Answer from the drawing. Dimensions are ordinates in mm from the lowest x, y and z of the part. Round coordinates to 2 decimals unless told otherwise and drop trailing zeros. Write each loop counter-clockwise with the first axis right and the second up, starting at its lowest first coordinate (ties: lowest second). Pieces come first, ordered by that corner, then holes. Notation, with made-up numbers: (5, 56.25) - (56, 56.25) arc R10 ccw to (56, 72.25) - close; hole circle Ø5 at (80, -24). An arc over 180 degrees is marked (long way). Answer in a Markdown table with one row per item.
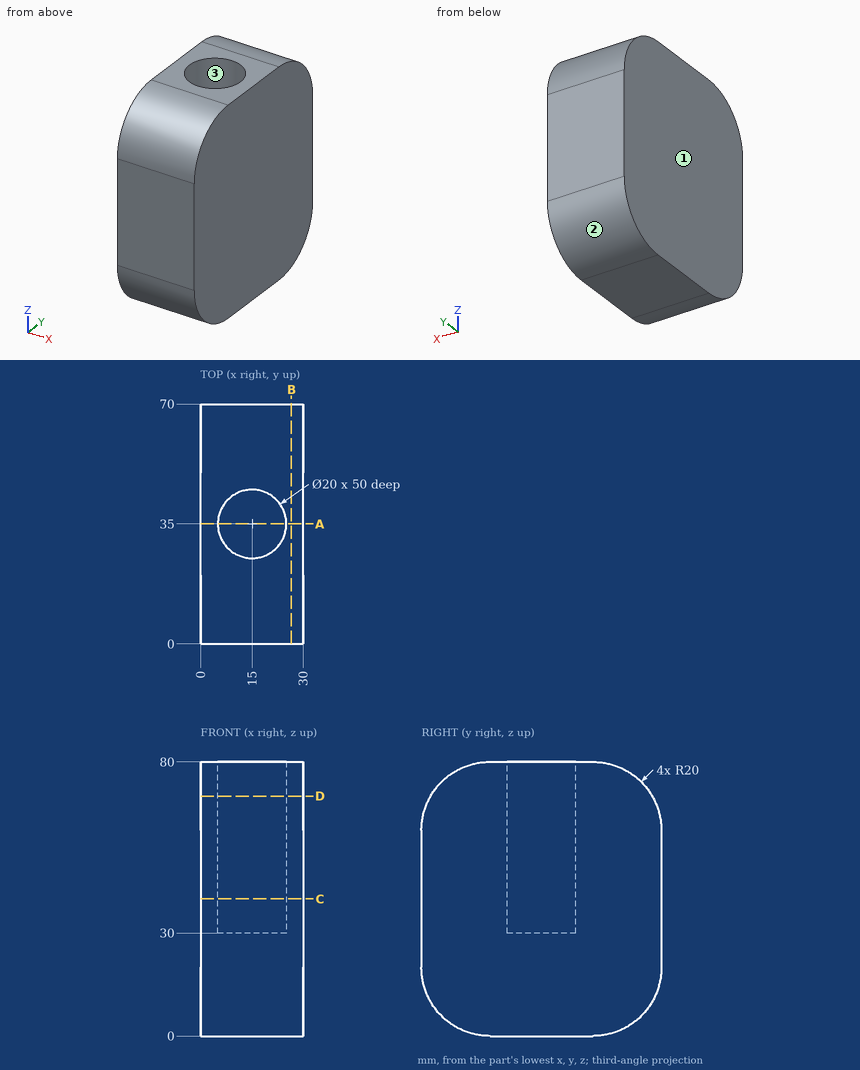
(1) Section D-D (z = 70) is taken. Give the vertices of the cut face in (x, y), and give its area (3 significant figures).
Checked values:
| item | result |
|---|---|
| outline | (0, 2.68) - (30, 2.68) - (30, 67.32) - (0, 67.32) - close; hole circle Ø20 at (15, 35) |
| area | 1,630 mm2 |
(2) For a pull along X with two mould halves and no side action, classify the marked faces 1, 2 and 3 as pulls with the +X half, pulls with the -X half, needs draft (parallel to the pull), parting line crosses it, or undercut.
Checked values:
| item | result |
|---|---|
| face 1 | pulls with the -X half |
| face 2 | needs draft |
| face 3 | undercut |
(3) Section B-B (x = 26.5) is taken. Give the vertices of the cut face in (y, z), and give its area (3 significant figures).
Checked values:
| item | result |
|---|---|
| outline | (0, 20) arc R20 ccw to (20, 0) - (50, 0) arc R20 ccw to (70, 20) - (70, 60) arc R20 ccw to (50, 80) - (20, 80) arc R20 ccw to (0, 60) - close |
| area | 5,260 mm2 |
(4) Find the intervals of material crossed by line 1 (Y direction, x = 15, z = 52); line 2 (Y direction, x = 11.5, z = 39); line 3 (X direction, y = 40.5, z = 59.5), in increasing order.
Checked values:
| item | result |
|---|---|
| line 1 | y = 0 to 25, 45 to 70 |
| line 2 | y = 0 to 25.63, 44.37 to 70 |
| line 3 | x = 0 to 6.65, 23.35 to 30 |
(5) Section A-A (y = 35) is taken. Give the vertices of the cut face in (x, z), and give its area (3 significant figures).
Checked values:
| item | result |
|---|---|
| outline | (0, 0) - (30, 0) - (30, 80) - (25, 80) - (25, 30) - (5, 30) - (5, 80) - (0, 80) - close |
| area | 1,400 mm2 |
(6) Flat-ended cylindrical pins translate along their axes: pin 1 (3 mm diameter, centred on x = 18, y = 11.5, fed in from -Z) (3 decimals); pin 2 (16 mm diameter, centred on x = 15, y = 35, fed in from +Z); pin 3 (6 mm diameter, centred on x = 19, z = 13, fed in from -Y). Find the tip coordinate at first contact, or state that the pin passes through.
Checked values:
| item | result |
|---|---|
| pin 1 | stops at z = 1.265 |
| pin 2 | stops at z = 30 |
| pin 3 | stops at y = 0.4 |
(7) Section C-C (z = 40) is taken. Give the vertices of the cut face in (x, y).
Checked values:
| item | result |
|---|---|
| outline | (0, 0) - (30, 0) - (30, 70) - (0, 70) - close; hole circle Ø20 at (15, 35) |
